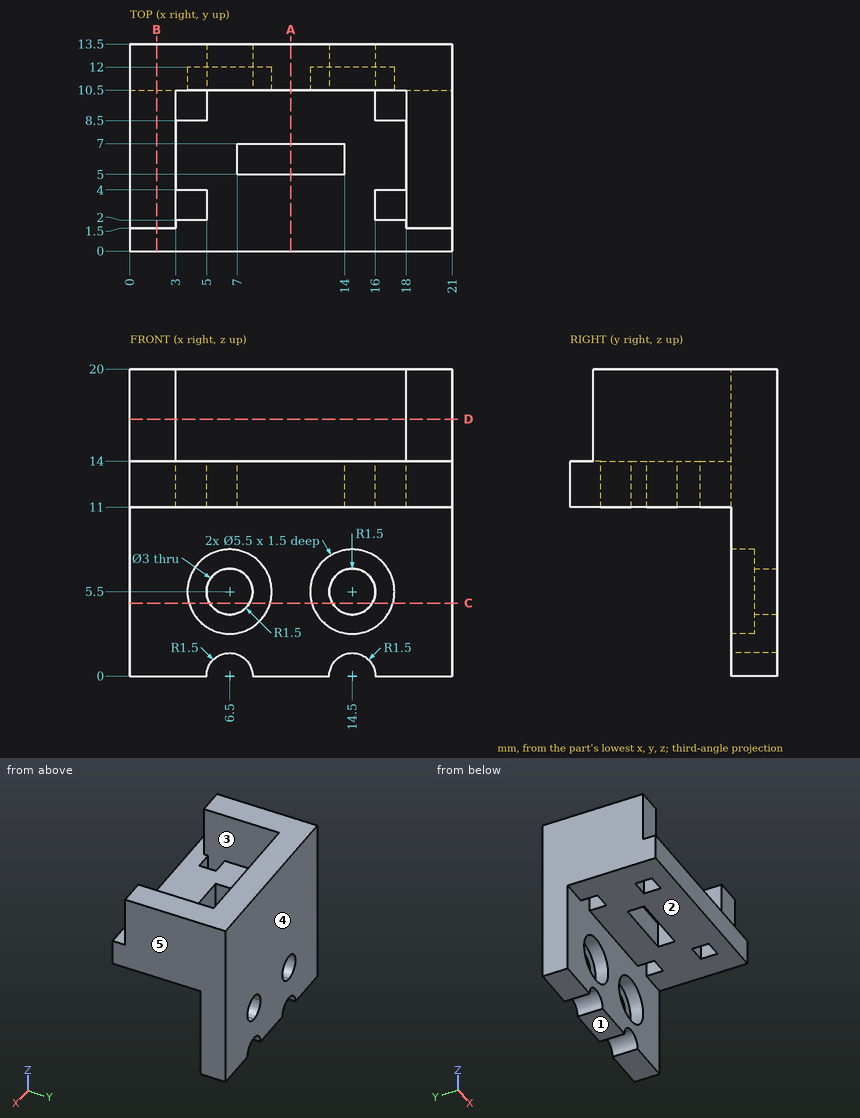
Part print with two shaded views. Sizes in mm from the minimum x, y, z corner. A direction names the side the tool comes from. Coordinates: 2 decimals unless noted, no trailing zeros. Order: outer loops, then holes, each group sorted by start corner. A loop starts at its lowest first (then second) coordinate and runs counter-clockwise, first axis right, second up. Notation, with made-up numbers: (32.25, -4.5) - (39.25, -4.5) arc R29 ccw to (39.25, 34.5) - close; hole circle Ø5 at (-11, -19). An arc over 180 degrees is marked (long way). Write item = value, one per line. Start each with the question number.
1) Saw through at C-C on z = 4.75. Write the cut outline in (x, y), then the cut area to 3 significant figures.
2) Saw through at B-B on x = 1.75. Write the cut outline in (y, z).
3) Saw through at D-D on z = 16.75. Write the cut outline in (x, y).
4) Two-plate mould, pull along X, no slides. Class the marked faces 3, 4 and 5: pulls with the +X half, pulls with the -X half, needs draft (parallel to the pull), parting line crosses it, or undercut.
5) Flat gauge pins, fed straight in: pin 1 Ø1.5 at (y, z) = (4, 12) entering from -X; pin 2 Ø6 at (x, z) = (15.5, 6) entering from -Y; pin 3 Ø3 at (x, y) = (15.5, 5.5) entering from -Z. Where does each tip first touch, or does it go through?
6) Saw through at A-A on x = 10.5. Write the cut outline in (y, z), then the cut area to 3 significant figures.
7) 3-axis set-ups, long thin cutter, end or side, ignore diameter. For the marked faces 1 and 2: which of +Z, -Z, +X, -X, +Y, -Y reach the whole face in a straight line?
8) Wall check: line 1 along Z through (x, y) = (6.5, 13.2); line 2 along X through (y, z) = (7.5, 17.5); line 3 along Z through (x, y) = (18.5, 2.75). Give the ranges that are in metal, low to high. Write a range as from..to.
From the geometry:
q1.outline = (0, 10.5) - (3.85, 10.5) - (3.85, 12) - (5.2, 12) - (5.2, 13.5) - (0, 13.5) - close; (7.8, 12) - (9.15, 12) - (9.15, 10.5) - (11.85, 10.5) - (11.85, 12) - (13.2, 12) - (13.2, 13.5) - (7.8, 13.5) - close; (15.8, 12) - (17.15, 12) - (17.15, 10.5) - (21, 10.5) - (21, 13.5) - (15.8, 13.5) - close
q1.area = 39.3 mm^2
q2.outline = (0, 11) - (10.5, 11) - (10.5, 0) - (13.5, 0) - (13.5, 20) - (1.5, 20) - (1.5, 14) - (0, 14) - close
q3.outline = (0, 1.5) - (3, 1.5) - (3, 10.5) - (18, 10.5) - (18, 1.5) - (21, 1.5) - (21, 13.5) - (0, 13.5) - close
q4.face_3 = undercut
q4.face_4 = needs draft
q4.face_5 = pulls with the +X half
q5.pin_1 = 0
q5.pin_2 = 10.5
q5.pin_3 = 11
q6.outline = (0, 11) - (5, 11) - (5, 14) - (0, 14) - close; (7, 11) - (10.5, 11) - (10.5, 0) - (13.5, 0) - (13.5, 20) - (10.5, 20) - (10.5, 14) - (7, 14) - close
q6.area = 85.5 mm^2
q7.face_1 = -Z, +X, -X, +Y, -Y
q7.face_2 = -Z, +X, -X, -Y
q8.line_1 = 1.5..4, 7..20
q8.line_2 = 0..3, 18..21
q8.line_3 = 11..20
